For this review, take the finished solid that the model builds, in its own axes (mm). A direction names the side the tool comes from. Coordinates: 2 decimals unless noted, no trailing zeros. Write each loop counter-clockwise with the first axis right and the second up, starting at its lowest first coordinate (ties: lowest second). Pieces come first, ordered by that corner, then holes.
1) Mouldability with a two-part tool opening along Y and no side actions: class faces 3 (the face through (-1.5, 0.07, -9.77)), 4 (the face through (0, 0, -20)), 5 (the face through (-0.86, -0.51, 1.06)) as pulls with the +Y half, pulls with the -Y half, needs draft (parallel to the pull), parting line crosses it, or undercut.
2) We need section A-A on z = -12.75. Write out the cut boundary in (x, y).
3) Insertion check: P1, Ø3, axis at x = 1, z = -7, coming from the +Y side; P2, Ø0.5, axis at x = 0, z = 1, coming from the -Y side; P3, Ø2, axis at y = 1.5, z = -13, coming from the -X side. Each pin has a flat end and moves straight along its axis. Give the tip position at first contact, or say it passes through.
4) To check wall thickness, follow line 1 along Z through (x, y) = (-1.1, -0.4); line 2 along X through (y, z) = (0.4, 0.5); line 3 along Z through (x, y) = (1.7, -1). State the ranges of each line that lie inside material, in increasing order.
5) For faces 1 (the face through (0, 2, 0)), 2 (the face through (0.86, 0.51, 1.06)), list the 3-axis set-ups (+Z, -Z, +X, -X, +Y, -Y) from which the entire face can be reached by the end or side of a thin tool; tool diameter is ignored.
Solid Edge part; units mm, degrees
sketch "Sketch1" plane through (0, 0, 0) normal (0, -1, 0) x (1, 0, 0)
  line L0 (0, -20) -> (1.5, -20)
  line L1 (1.5, -20) -> (1.5, -0.115)
  arc A0 (1.5, -0.105) -> (1.5, -0.115) centre (1.5038, -0.11) ccw
  line L2 (1.5, -0.105) -> (1.5, 0)
  line L3 (1.5, 0) -> (2.85, 0)
  line L4 (2.85, 0) -> (2.85, 0.165)
  arc A1 (1.27, 1.65) -> (2.85, 0.165) centre (-0.3628, -1.6703) cw
  line L5 (0, 1.65) -> (1.27, 1.65)
  dimension "D1" = 1.5
revolve "RevolvedProtrusion1" add sketch "Sketch1" angle 360 about axis through (0, 0, 5) along (0, 0, -1)
sketch "Sketch2" plane through (0, 0, 0) normal (0, -1, 0) x (1, 0, 0)
  line L0 (0, -0.0566) -> (1.1545, 0.61)
  line L1 (1.1545, 0.61) -> (1.1545, 1.65)
  line L2 (1.1545, 1.65) -> (0, 1.65)
revolve "RevolvedCutout1" cut sketch "Sketch2" angle 360 about axis through (0, 0, 5.3) along (0, 0, -1)
sketch "Sketch3" plane through (0, 0, 0) normal (0, 0, -1) x (0, 1, 0)
  arc A0 (-1, 0.577) -> (-1, -0.577) centre (0, 0) ccw
  line L0 (-1, 0.577) -> (-1, -0.577)
extrude "Protrusion1" add sketch "Sketch3" against normal blind 1.65
pattern_circular "Pattern1" count 6 over 360 about axis through (0, 0, 0) along (0, 0, -1) of "Protrusion1"
fillet "Round_1" radius 0.185 1 edges at (-1.27, 0, 1.65)
sketch "Sketch4" plane through (0, 0, 0) normal (0, -1, 0) x (1, 0, 0)
  line L0 (0, 0.9501) -> (1.2122, 1.65)
  line L1 (1.2122, 1.65) -> (0, 1.65)
revolve "RevolvedCutout2" cut sketch "Sketch4" angle 360 about axis through (0, 0, 5.3) along (0, 0, -1)
sketch "Sketch5" plane through (0, 0, 0) normal (0, -1, 0) x (1, 0, 0)
  line L0 (-1.5, 0) -> (-1.5, -0.1)
  line L1 (-1.6, 0) -> (-1.5, 0)
  arc A0 (-1.6, 0) -> (-1.5, -0.1) centre (-1.6, -0.1) cw
revolve "RevolvedProtrusion2" add sketch "Sketch5" angle 360 about axis through (0, 0, -0.5) along (0, 0, 1)
cosmetic_thread "Thread1"
chamfer "Chamfer1" distance 0.3065 angle 45 1 edges at (-1.5, 0, -20)
properties material "Stahl"
Result:
1. face 3: parting line crosses it
1. face 4: needs draft
1. face 5: undercut
2. outline: circle Ø3 at (0, 0)
3. P1: stops at y = 1.5
3. P2: stops at y = -2.44
3. P3: stops at x = -1.41
4. line 1: z = -20 to 1.63
4. line 2: x = -2.6 to -0.88, 0.88 to 2.6
4. line 3: z = 0 to 1.2
5. face 1: -Z
5. face 2: +Z
